The model under review builds one solid part; all positions refer to its coordinate system, in mm. Round coordinates to 2 decimals unless told otherwise and drop trailing zeros. Write each loop counter-clockwise with the first axis right and the second up, starting at its lowest first coordinate (ties: lowest second). Pieces come first, ordered by that corner, then holes.
Item 1: To check wall thickness, follow L1, parallel to Y at x = 115, z = 16.75; L2, parallel to Y at x = 118.5, z = 18.5; L3, parallel to X at y = 18.5, z = 18.75. State the ranges of each line that lie inside material, in increasing order.
Item 2: Clearance check with flat-ended pins moving along their axes: pin 1 Ø3 at (y, z) = (-13.5, 14.5) entering from +X; pin 2 Ø5 at (y, z) = (-53, 16.5) entering from +X; pin 3 Ø5 at (y, z) = (-28, 17.5) entering from +X. State where each tip first meets the part, or that it passes through.
Item 3: Add section A-A (z = 10). Give the boundary of the cut face in (x, y).
Item 4: Draft analysis for pull direction Y (two halves, no side actions). For faces 1 (the face through (131.997, 100.721, 0.301)), 2 (the face through (132.05, -109.91, 0.3)), 3 (the face through (35.024, -6.825, 9.874)), state which applies: +Y half, -Y half, draft (parallel to the pull), parting line (faces both ways), or undercut.
```python
from build123d import *

# Parameters (mm, degrees)
BOSS_EXTRUDE1_DEPTH = 20
FILLET1_R           = 1


with BuildPart() as part:
    # Sketch2 → Boss-Extrude1 (new body)
    with BuildSketch(Plane.XY):
        with BuildLine():
            Line((0, 105.351887556), (0, -114.648112444))
            Line((0, -114.648112444), (130, -114.648112444))
            Line((130, -114.648112444), (135, -104.648112444))
            ThreePointArc((135, -104.648112444), (35, -4.648112444), (135, 95.351887556))
            Line((135, 95.351887556), (130, 105.351887556))
            Line((130, 105.351887556), (0, 105.351887556))
        make_face()
    extrude(amount=BOSS_EXTRUDE1_DEPTH)

    # Fillet1
    fillet1_edges = [part.edges().sort_by_distance(p)[0] for p in [
        (130, 105.351887556, 10),
        (135, 95.351887556, 10),
        (135, -104.648112444, 10),
        (130, -114.648112444, 10),
        (0, -114.648112444, 10),
        (0, 105.351887556, 10),
        (65, -114.648112444, 20),
        (132.5, -109.648112444, 20),
        (35, -4.648112444, 20),
        (132.5, 100.351887556, 20),
        (65, 105.351887556, 20),
        (132.5, 100.351887556, 0),
        (35, -4.648112444, 0),
        (132.5, -109.648112444, 0),
        (65, -114.648112444, 0),
        (0, -4.648112444, 0),
        (65, 105.351887556, 0),
        (0, -4.648112444, 20),
    ]]
    fillet(fillet1_edges, radius=FILLET1_R)


solid = part.part
```
Numbers:
1. L1: y = -114.65 to -102.63, 93.33 to 105.35
1. L2: y = -114.65 to -103.28, 93.98 to 105.35
1. L3: x = 0 to 37.72
2. pin 1: stops at x = 35.54
2. pin 2: stops at x = 48.89
2. pin 3: stops at x = 38.4
3. outline: (0, -113.65) arc R1 ccw to (1, -114.65) - (129.38, -114.65) arc R1 ccw to (130.28, -114.1) - (134.28, -106.08) arc R1 ccw to (133.4, -104.64) arc R100 cw to (133.4, 95.34) arc R1 ccw to (134.28, 96.79) - (130.28, 104.8) arc R1 ccw to (129.38, 105.35) - (1, 105.35) arc R1 ccw to (0, 104.35) - close
4. face 1: +Y half
4. face 2: -Y half
4. face 3: undercut
